```python
from build123d import *

# Parameters (mm, degrees)
BOSS_EXTRUDE1_DEPTH = 5
SKETCH2_W           = 213.862691863
SKETCH2_H           = 54.913039258
CUT_EXTRUDE1_DEPTH  = 5
BOSS_EXTRUDE2_DEPTH = 29
SKETCH4_W           = 6
SKETCH4_H           = 6
BOSS_EXTRUDE3_DEPTH = 30
SKETCH5_W           = 6
SKETCH5_H           = 6
BOSS_EXTRUDE4_DEPTH = 30
FILLET1_R           = 10
SKETCH7_R           = 2
CUT_EXTRUDE2_DEPTH  = 29
SKETCH8_W           = 20
SKETCH8_H           = 20
CUT_EXTRUDE3_DEPTH  = 10


# Read off the part's stored shape, not the designer's step: Boss-Extrude2
with BuildPart() as part:
    # Sketch1 → Boss-Extrude1 (new body)
    with BuildSketch(Plane(origin=(0, 0, 0), x_dir=(1, 0, 0), z_dir=(0, 1, 0))):
        with BuildLine():
            Line((0, 130), (0, 0))
            Line((0, 0), (210, 0))
            Line((210, 0), (210, 130))
            ThreePointArc((210, 130), (105, 25), (0, 130))
        make_face()
        with BuildLine():
            ThreePointArc((210, 130), (105, 235), (0, 130))
            Line((0, 130), (210, 130))
        make_face()
        with BuildLine():
            Line((210, 130), (0, 130))
            ThreePointArc((0, 130), (105, 25), (210, 130))
        make_face()
    extrude(amount=BOSS_EXTRUDE1_DEPTH)

    # Sketch2 → Cut-Extrude1 (cut)
    with BuildSketch(Plane(origin=(0, 5, 0), x_dir=(1, 0, 0), z_dir=(0, 1, 0))):
        with Locations((106.931345932, 241.686519629)):
            Rectangle(SKETCH2_W, SKETCH2_H)
    extrude(amount=-CUT_EXTRUDE1_DEPTH, mode=Mode.SUBTRACT)

    # Boss-Extrude2 outline → Boss-Extrude2 (add)
    with BuildSketch(Plane(origin=(0, 0, 0), x_dir=(-1, 0, 0), z_dir=(0, -1, 0))):
        with BuildLine():
            ThreePointArc((-50.307838608, 214.23), (-44.96798765, 206.685226506), (-36.076936839, 209.212444505))
            ThreePointArc((-36.076936839, 209.212444505), (-39.144584131, 211.78058572), (-42.307838608, 214.23))
            Line((-42.307838608, 214.23), (-50.307838608, 214.23))
        make_face()
        with BuildLine():
            Line((0, 0), (0, 10))
            ThreePointArc((0, 10), (-7.071067812, 7.071067812), (-10, 0))
            Line((-10, 0), (0, 0))
        make_face()
        with BuildLine():
            ThreePointArc((-173.923063161, 209.212444505), (-165.03201235, 206.685226506), (-159.692161392, 214.23))
            Line((-159.692161392, 214.23), (-167.692161392, 214.23))
            ThreePointArc((-167.692161392, 214.23), (-170.855415869, 211.78058572), (-173.923063161, 209.212444505))
        make_face()
        with BuildLine():
            Line((-210, 0), (-200, 0))
            ThreePointArc((-200, 0), (-202.928932188, 7.071067812), (-210, 10))
            Line((-210, 10), (-210, 0))
        make_face()
    extrude(amount=BOSS_EXTRUDE2_DEPTH)

    # Sketch4 → Boss-Extrude3 (add)
    with BuildSketch(Plane.XZ):
        with Locations((171, -87)):
            Rectangle(SKETCH4_W, SKETCH4_H)
    extrude(amount=BOSS_EXTRUDE3_DEPTH)

    # Sketch5 → Boss-Extrude4 (add)
    with BuildSketch(Plane(origin=(0, 0, 0), x_dir=(-1, 0, 0), z_dir=(0, -1, 0))):
        with Locations((-72, 112)):
            Rectangle(SKETCH5_W, SKETCH5_H)
    extrude(amount=BOSS_EXTRUDE4_DEPTH)

    # Fillet1
    fillet1_edges = [part.edges().sort_by_distance(p)[0] for p in [
        (168, 0, -87),
        (171, 0, -90),
        (174, 0, -87),
        (171, 0, -84),
        (75, 0, -112),
        (72, 0, -109),
        (69, 0, -112),
        (72, 0, -115),
    ]]
    fillet(fillet1_edges, radius=FILLET1_R)

    # Sketch7 → Cut-Extrude2 (cut)
    with BuildSketch(Plane(origin=(0, 5, 0), x_dir=(1, 0, 0), z_dir=(0, 1, 0))):
        with Locations(Location((61.329013771, 105, 0), (0, 0, 270))):
            Circle(SKETCH7_R)
        with Locations(Location((103.829013771, 62.5, 0), (0, 0, 270))):
            Circle(SKETCH7_R)
        with Locations(Location((103.829013771, 147.5, 0), (0, 0, 270))):
            Circle(SKETCH7_R)
        with Locations(Location((146.329013771, 105, 0), (0, 0, 270))):
            Circle(SKETCH7_R)
    extrude(amount=-CUT_EXTRUDE2_DEPTH, mode=Mode.SUBTRACT)

    # Sketch8 → Cut-Extrude3 (cut)
    with BuildSketch(Plane(origin=(0, 5, 0), x_dir=(1, 0, 0), z_dir=(0, 1, 0))):
        with Locations((154.091797389, 63.651218277)):
            Rectangle(SKETCH8_W, SKETCH8_H)
    extrude(amount=-CUT_EXTRUDE3_DEPTH, mode=Mode.SUBTRACT)


solid = part.part
```
For this review, take the finished solid that the model builds, in its own axes (mm). A direction names the side the tool comes from. Coordinates: 2 decimals unless noted, no trailing zeros. Loops run counter-clockwise (first coordinate to the right, second up) from the corner with the lowest first, then second, coordinate; pieces in that order, holes last. Notation, with made-up numbers: (63, 15) - (110, 15) arc R3 cw to (110, 19) - close; hole circle Ø6 at (-27, 6). An arc over 180 degrees is marked (long way). Use one line per item in the form item = value. Start each with the question number.
1) Take a section at C-C (y = -3.5). State the section outline as (x, z) points, plus the area to 3 significant figures.
2) Take a section at B-B (z = -80.5). State the section outline as (x, y) points.
3) Take a section at A-A (y = -18). State the section outline as (x, z) points, plus the area to 3 significant figures.
4) To check wall thickness, follow probe 1 along X at (y, z) = (1.15, -105); probe 2 along X at (y, z) = (2.35, -62.5); probe 3 along X at (y, z) = (3.5, -56). State the ranges of each line that lie inside material, in increasing order. Write a range as from..to.
5) Take a section at D-D (x = 131.5). State the section outline as (y, z) points.
6) For faces 1 (the face through (168, -20, -87)), 2 (the face through (154, 3, -53.651)), 3 (the face through (171, -2, -94)), list the 3-axis set-ups (+Z, -Z, +X, -X, +Y, -Y) from which the entire face can be reached by the end or side of a thin tool; tool diameter is ignored.
7) For pin 1 (5 mm diameter, centred on x = 103.83, z = -62.5, fed in from +Y); pin 2 (10 mm diameter, centred on x = 63, z = -121.5, fed in from -Y); pin 3 (6.5 mm diameter, centred on y = -22, z = -113, fed in from -X); pin 4 (2 mm diameter, centred on x = 80.5, y = -3, fed in from +Z), all flat-tipped, find the tip position at first contact; note any pin that passes through.
8) Draft analysis for pull direction Z (two halves, no side actions). For faces 4 (the face through (165.16, -14.3, -206.64)), 5 (the face through (171, -20, -90)), 6 (the face through (206, -29, -4)), 7 (the face through (105, 2, 0)), state which applies: released by +Z, released by -Z, zero draft, split by the parting line, or undercut.
From the geometry:
q1.outline = (0, -10) arc R10 ccw to (10, 0) - (0, 0) - close; (36.08, -209.21) arc R105 ccw to (42.31, -214.23) - (50.31, -214.23) arc R8 ccw to start; (66.6, -117.4) - (77.4, -117.4) - (77.4, -106.6) - (66.6, -106.6) - close; (159.69, -214.23) - (167.69, -214.23) arc R105 ccw to (173.92, -209.21) arc R8 ccw to start; (165.6, -92.4) - (176.4, -92.4) - (176.4, -81.6) - (165.6, -81.6) - close; (200, 0) arc R10 ccw to (210, -10) - (210, 0) - close
q1.area = 549 mm2
q2.outline = (0, 0) - (158, 0) arc R10 cw to (164.5, -2.4) - (177.5, -2.4) arc R10 cw to (184, 0) - (210, 0) - (210, 5) - (0, 5) - close
q3.outline = (0, -10) arc R10 ccw to (10, 0) - (0, 0) - close; (36.08, -209.21) arc R105 ccw to (42.31, -214.23) - (50.31, -214.23) arc R8 ccw to start; (69, -115) - (75, -115) - (75, -109) - (69, -109) - close; (159.69, -214.23) - (167.69, -214.23) arc R105 ccw to (173.92, -209.21) arc R8 ccw to start; (168, -90) - (174, -90) - (174, -84) - (168, -84) - close; (200, 0) arc R10 ccw to (210, -10) - (210, 0) - close
q3.area = 388 mm2
q4.probe_1 = 0..59.33, 63.33..144.33, 148.33..210
q4.probe_2 = 0..101.83, 105.83..144.09, 164.09..210
q4.probe_3 = 0..144.09, 164.09..210
q5.outline = (0, -214.23) - (5, -214.23) - (5, 0) - (0, 0) - close
q6.face_1 = +Z, -X, -Y
q6.face_2 = +Y, -Y
q6.face_3 = +X, -X, -Y
q7.pin_1 = 5
q7.pin_2 = -3.14
q7.pin_3 = 69
q7.pin_4 = through
q8.face_4 = undercut
q8.face_5 = undercut
q8.face_6 = zero draft
q8.face_7 = released by +Z
